Source: three-view drawing plus pictorial views. Frame: mm from the lowest corner of the part. A direction names the side the tool comes from. Round coordinates to 2 decimals unless told otherwise and drop trailing zeros. Loops run counter-clockwise (first coordinate to the right, second up) from the corner with the lowest first, then second, coordinate; pieces in that order, holes last. Notation, with made-up numbers: (-3, -23) -> (12, -23) arc R34 ccw to (12, 10) -> close; hole circle Ø7 at (-24, 27.5). An arc over 180 degrees is marked (long way). Answer as a JSON object with one key per item and string values. Group by question number.
Item 1: Section query B-B on x = 4.5. Return loops of the section in (y, z), and give its area (3 significant figures).
Item 2: Set-up query: the marked faces 4 and 5. Return all of +Z, -Z, +X, -X, +Y, -Y with unobstructed straight access to the full face (end or side cutting, diameter ignored); none if empty.
Item 3: Section query A-A on z = 4.5. Return loops of the section in (x, y), and give its area (3 significant figures).
Item 4: Section query D-D on z = 7.75. Return loops of the section in (x, y), and give its area (3 significant figures).
Item 5: Material intervals for line 1 (Y direction, x = 0.5, z = 6.5); line 2 (X direction, y = 2.05, z = 4.5), sorted ascending. Write a range as [from, to].
Item 6: Section query C-C on y = 3.45. Return loops of the section in (x, z), and give its area (3 significant figures).
Item 7: Draft query along Y for the marked faces 1, 2 and 3. Return one class per face: released by +Y, released by -Y, zero draft, split by the parting line, or undercut.
Item 8: Pin query (flat end, axial travel): pin 1 (1 mm diameter, centred on x = 5, z = 2.5, fed in from -Y); pin 2 (4.5 mm diameter, centred on x = 3.5, z = 5.5, fed in from +Y); pin 3 (2 mm diameter, centred on x = 7, y = 3, fed in from +Z); pin 4 (2 mm diameter, centred on x = 4.5, y = 2, fed in from +Z). Return the tip coordinate at first contact, or that it passes through.
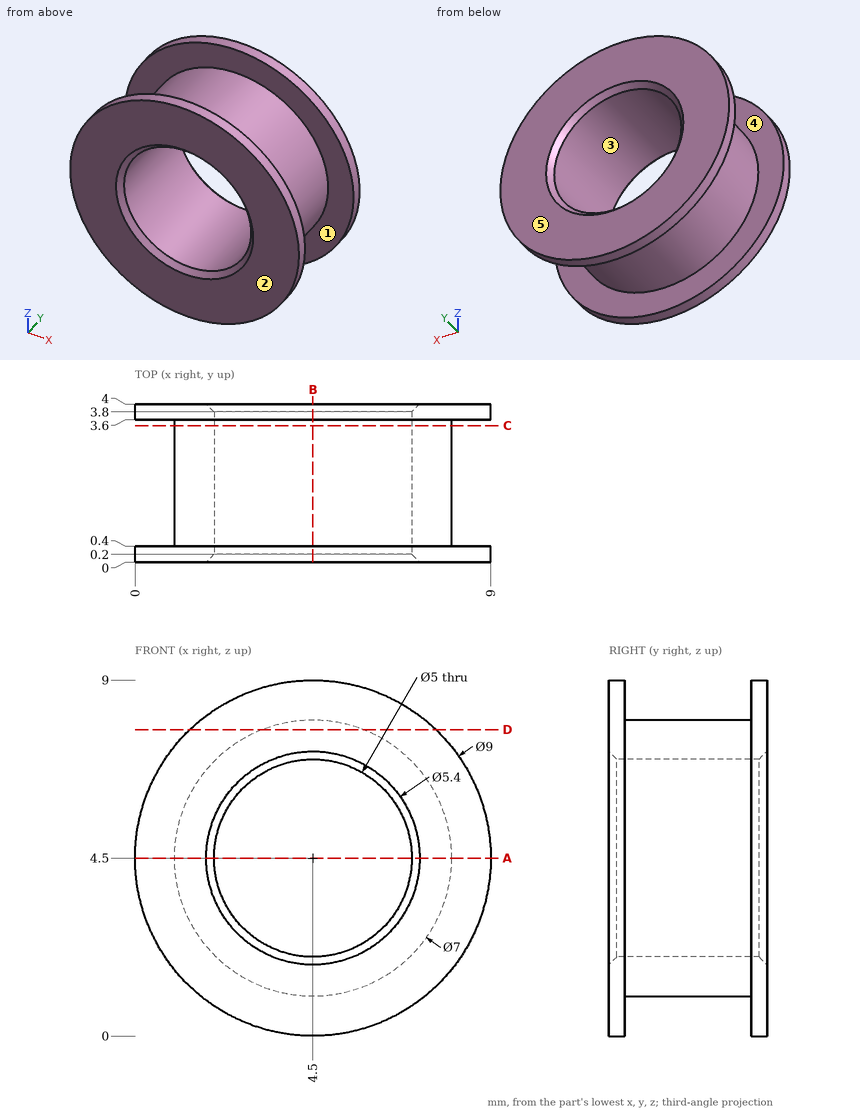
Solved:
{
 "1": {"outline": "(0, 0) -> (0.4, 0) -> (0.4, 1) -> (3.6, 1) -> (3.6, 0) -> (4, 0) -> (4, 1.8) -> (3.8, 2) -> (0.2, 2) -> (0, 1.8) -> close; (0, 7.2) -> (0.2, 7) -> (3.8, 7) -> (4, 7.2) -> (4, 9) -> (3.6, 9) -> (3.6, 8) -> (0.4, 8) -> (0.4, 9) -> (0, 9) -> close", "area": "9.52 mm²"},
 "2": {"face 4": "none", "face 5": "+Z, -Z, +X, -X, +Y"},
 "3": {"outline": "(0, 0) -> (1.8, 0) -> (2, 0.2) -> (2, 3.8) -> (1.8, 4) -> (0, 4) -> (0, 3.6) -> (1, 3.6) -> (1, 0.4) -> (0, 0.4) -> close; (7, 0.2) -> (7.2, 0) -> (9, 0) -> (9, 0.4) -> (8, 0.4) -> (8, 3.6) -> (9, 3.6) -> (9, 4) -> (7.2, 4) -> (7, 3.8) -> close", "area": "9.52 mm²"},
 "4": {"outline": "(1.39, 0) -> (7.61, 0) -> (7.61, 0.4) -> (5.8, 0.4) -> (5.8, 3.6) -> (7.61, 3.6) -> (7.61, 4) -> (1.39, 4) -> (1.39, 3.6) -> (3.2, 3.6) -> (3.2, 0.4) -> (1.39, 0.4) -> close", "area": "13.3 mm²"},
 "5": {"line 1": "[0, 0.4], [3.6, 4]", "line 2": "[1, 2], [7, 8]"},
 "6": {"outline": "circle Ø7 at (4.5, 4.5); hole circle Ø5 at (4.5, 4.5)", "area": "18.8 mm²"},
 "7": {"face 1": "undercut", "face 2": "released by -Y", "face 3": "zero draft"},
 "8": {"pin 1": "y = 0.14", "pin 2": "y = 4", "pin 3": "z = 8.67", "pin 4": "z = 8"}
}
